Check sheet for the modelled part. Datum: model origin and axes. Units: mm. Face numbers are marked on the shaded views. Coordinates: 2 decimals unless noted, no trailing zeros. Loops run counter-clockwise (first coordinate to the right, second up) from the corner with the lowest first, then second, coordinate; pieces in that order, holes last. Notation, with made-up numbers: (-6.75, 76.25) - (-1.75, 76.25) arc R19 ccw to (-1.75, 111.25) - close; hole circle Ø10 at (77.5, 3). An arc over 180 degrees is marked (long way). Use a Markdown table: item, result. Add a question column.
1) Draft check along X on the marked faces 1, 2 and 3. Enter one of: pulls with the +X half, pulls with the -X half, needs draft (parallel to the pull), parting line crosses it, or undercut.
2) Thickness scan on line 1 (Y direction, x = -4, z = 0); line 2 (X direction, y = 1.8, z = 0); line 3 (Z direction, x = 9, y = 35). Record the ranges inside material, lowest first.
3) Sectioned sample at A-A, the plane y = 19. Enter the section's corners in (x, z), then the cut area to 3 significant figures.
4) Go/stop test with flat-tipped pins: P1, Ø10, axis at y = 22.5, z = 4, coming from the -X side; P2, Ø3, axis at x = 12, y = 23.5, coming from the +Z side; P3, Ø4.5, axis at x = -3, z = 0.5, coming from the -Y side. Record where each tip stops, or that it passes through.
from build123d import *

# Parameters (mm, degrees)
SKETCH3_R          = 2.5
CUT_EXTRUDE1_DEPTH = 1
FILLET1_R          = 5
SCALE1_SCALE       = 3


# Read off the part's stored shape, not the designer's step: Boundary1
with BuildPart() as part:
    # Boundary1 outline → Boundary1 (revolve)
    with BuildSketch(Plane.XY):
        Polygon((0, 0), (5, 0), (7.5, 15), (0, 15), align=None)
    revolve(axis=Axis((0, 0, 0), (0, 1, 0)))

    # Sketch3 → Cut-Extrude1 (cut)
    with BuildSketch(Plane.XZ):
        with Locations(Location((0, 0, 0), (0, 0, 270))):
            Circle(SKETCH3_R)
    extrude(amount=-CUT_EXTRUDE1_DEPTH, mode=Mode.SUBTRACT)

    # Fillet1
    fillet1_edges = [part.edges().sort_by_distance(p)[0] for p in [
        (-7.5, 15, 0),
    ]]
    fillet(fillet1_edges, radius=FILLET1_R)


with BuildPart() as part_1:
    # Scale1: scaled about (0, 0, 0)
    add(part.part.scale(SCALE1_SCALE))


solid = part_1.part
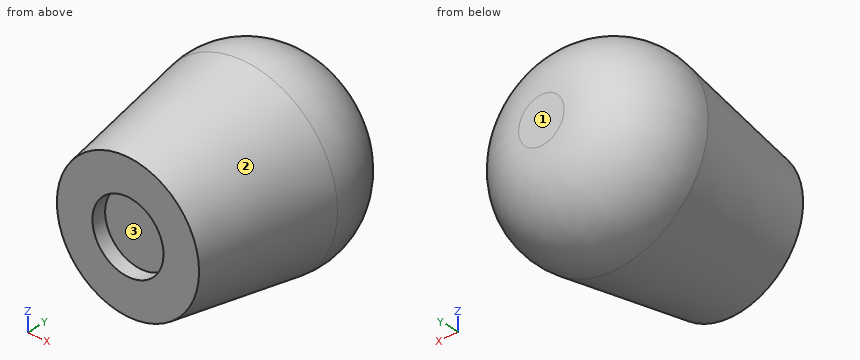
Solved:
| question | item | result |
|---|---|---|
| 1 | face 1 | needs draft |
| 1 | face 2 | parting line crosses it |
| 1 | face 3 | undercut |
| 2 | line 1 | y = 3 to 45 |
| 2 | line 2 | x = -15.3 to -7.5, 7.5 to 15.3 |
| 2 | line 3 | z = -16.66 to 16.66 |
| 3 | outline | circle Ø36.33 at (0, 0) |
| 3 | area | 1,040 mm2 |
| 4 | P1 | stops at x = -19.42 |
| 4 | P2 | stops at z = 15.78 |
| 4 | P3 | stops at y = 3 |
